Verification items for the finished model (mm, model axes). Round coordinates to 2 decimals unless told otherwise and drop trailing zeros. Write each loop counter-clockwise with the first axis right and the second up, starting at its lowest first coordinate (ties: lowest second). Pieces come first, ordered by that corner, then holes. Notation, with made-up numbers: (-5, 3) - (25, 3) arc R16 ccw to (25, 11) - close; hole circle Ø6 at (-19.5, -27.5). An arc over 180 degrees is marked (long way). Answer as a JSON object with one key per item and string values. Group by question number.
1) Section check C-C (z = 16.5). Enter the section's corners in (x, y).
2) Section check B-B (x = 0). Enter the section's corners in (y, z).
3) Go/stop test with flat-tipped pins: pin 1 Ø1.8 at (x, z) = (12.73, 12.73) entering from -Y; pin 2 Ø0.8 at (y, z) = (0.5, 9.5) entering from -X; pin 3 Ø0.8 at (y, z) = (0.5, 11) entering from +X; pin 4 Ø3.5 at (x, z) = (-4.66, 17.39) entering from +Y. Record where each tip stops, or that it passes through.
4) Section check A-A (z = 0). Enter the section's corners in (x, y), then the cut area to 3 significant figures.
5) Thickness scan on line 1 (Z direction, x = -0.5, y = 1.2); line 2 (X direction, y = 0.2, z = -11.5); line 3 (X direction, y = 1.2, z = -8.5). Record the ranges inside material, lowest first.
```python
from build123d import *

# Parameters (mm, degrees)
SKETCH1_R           = 21
SKETCH1_R_2         = 1.5
SKETCH1_R_3         = 4.4
BOSS_EXTRUDE1_DEPTH = 1.5


with BuildPart() as part:
    # Sketch1 → Boss-Extrude1 (new body)
    with BuildSketch(Plane(origin=(0, 0, 0), x_dir=(1, 0, 0), z_dir=(0, 1, 0))):
        with Locations(Location((0, 0, 0), (0, 0, 270))):
            Circle(SKETCH1_R)
        with Locations(Location((-8, 0, 0), (0, 0, 270))):
            Circle(SKETCH1_R_2, mode=Mode.SUBTRACT)
        with Locations(Location((8, 0, 0), (0, 0, 270))):
            Circle(SKETCH1_R_2, mode=Mode.SUBTRACT)
        with Locations(Location((0, 9.5, 0), (0, 0, 270))):
            Circle(SKETCH1_R_2, mode=Mode.SUBTRACT)
        with Locations(Location((0, -9.5, 0), (0, 0, 270))):
            Circle(SKETCH1_R_2, mode=Mode.SUBTRACT)
        with Locations(Location((-12.727922061, 12.727922061, 0), (0, 0, 270))):
            Circle(SKETCH1_R_2, mode=Mode.SUBTRACT)
        with Locations(Location((4.658742812, 17.386664873, 0), (0, 0, 270))):
            Circle(SKETCH1_R_2, mode=Mode.SUBTRACT)
        with Locations(Location((17.386664873, 4.658742812, 0), (0, 0, 270))):
            Circle(SKETCH1_R_2, mode=Mode.SUBTRACT)
        with Locations(Location((12.727922061, -12.727922061, 0), (0, 0, 270))):
            Circle(SKETCH1_R_2, mode=Mode.SUBTRACT)
        with Locations(Location((-4.658742812, -17.386664873, 0), (0, 0, 270))):
            Circle(SKETCH1_R_2, mode=Mode.SUBTRACT)
        with Locations(Location((0, 0, 0), (0, 0, 270))):
            Circle(SKETCH1_R_3, mode=Mode.SUBTRACT)
        with Locations(Location((-17.386664873, -4.658742812, 0), (0, 0, 270))):
            Circle(SKETCH1_R_2, mode=Mode.SUBTRACT)
        with BuildLine():
            Line((-8.660254038, 3), (-12, 3))
            ThreePointArc((-12, 3), (-13.664100589, 3.890599608), (-13.846153846, 5.769230769))
            ThreePointArc((-13.846153846, 5.769230769), (-10.606601718, 10.606601718), (-5.769230769, 13.846153846))
            ThreePointArc((-5.769230769, 13.846153846), (-3.890599608, 13.664100589), (-3, 12))
            Line((-3, 12), (-3, 8.660254038))
            ThreePointArc((-3, 8.660254038), (-3.267949192, 7.660254038), (-4, 6.92820323))
            ThreePointArc((-4, 6.92820323), (-5.656854249, 5.656854249), (-6.92820323, 4))
            ThreePointArc((-6.92820323, 4), (-7.660254038, 3.267949192), (-8.660254038, 3))
        make_face(mode=Mode.SUBTRACT)
        with BuildLine():
            Line((-8.660254038, -3), (-12, -3))
            ThreePointArc((-12, -3), (-13.664100589, -3.890599608), (-13.846153846, -5.769230769))
            ThreePointArc((-13.846153846, -5.769230769), (-10.606601718, -10.606601718), (-5.769230769, -13.846153846))
            ThreePointArc((-5.769230769, -13.846153846), (-3.890599608, -13.664100589), (-3, -12))
            Line((-3, -12), (-3, -8.660254038))
            ThreePointArc((-3, -8.660254038), (-3.267949192, -7.660254038), (-4, -6.92820323))
            ThreePointArc((-4, -6.92820323), (-5.656854249, -5.656854249), (-6.92820323, -4))
            ThreePointArc((-6.92820323, -4), (-7.660254038, -3.267949192), (-8.660254038, -3))
        make_face(mode=Mode.SUBTRACT)
        with BuildLine():
            Line((3, 8.660254038), (3, 12))
            ThreePointArc((3, 12), (3.890599608, 13.664100589), (5.769230769, 13.846153846))
            ThreePointArc((5.769230769, 13.846153846), (10.606601718, 10.606601718), (13.846153846, 5.769230769))
            ThreePointArc((13.846153846, 5.769230769), (13.664100589, 3.890599608), (12, 3))
            Line((12, 3), (8.660254038, 3))
            ThreePointArc((8.660254038, 3), (7.660254038, 3.267949192), (6.92820323, 4))
            ThreePointArc((6.92820323, 4), (5.656854249, 5.656854249), (4, 6.92820323))
            ThreePointArc((4, 6.92820323), (3.267949192, 7.660254038), (3, 8.660254038))
        make_face(mode=Mode.SUBTRACT)
        with BuildLine():
            Line((8.660254038, -3), (12, -3))
            ThreePointArc((12, -3), (13.664100589, -3.890599608), (13.846153846, -5.769230769))
            ThreePointArc((13.846153846, -5.769230769), (10.606601718, -10.606601718), (5.769230769, -13.846153846))
            ThreePointArc((5.769230769, -13.846153846), (3.890599608, -13.664100589), (3, -12))
            Line((3, -12), (3, -8.660254038))
            ThreePointArc((3, -8.660254038), (3.267949192, -7.660254038), (4, -6.92820323))
            ThreePointArc((4, -6.92820323), (5.656854249, -5.656854249), (6.92820323, -4))
            ThreePointArc((6.92820323, -4), (7.660254038, -3.267949192), (8.660254038, -3))
        make_face(mode=Mode.SUBTRACT)
    extrude(amount=BOSS_EXTRUDE1_DEPTH)


solid = part.part
```
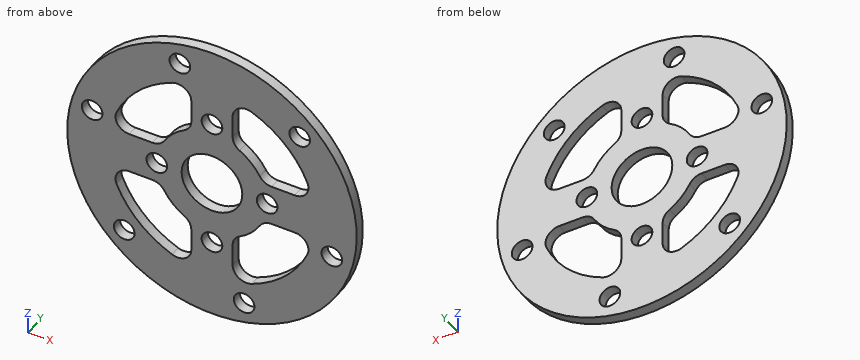
Returned:
{
 "1": {"outline": "(-12.99, 0) - (-5.87, 0) - (-5.87, 1.5) - (-12.99, 1.5) - close; (-3.45, 0) - (12.99, 0) - (12.99, 1.5) - (-3.45, 1.5) - close"},
 "2": {"outline": "(0, -21) - (1.5, -21) - (1.5, -11) - (0, -11) - close; (0, -8) - (1.5, -8) - (1.5, -4.4) - (0, -4.4) - close; (0, 4.4) - (1.5, 4.4) - (1.5, 8) - (0, 8) - close; (0, 11) - (1.5, 11) - (1.5, 21) - (0, 21) - close"},
 "3": {"pin 1": "through", "pin 2": "x = -18.93", "pin 3": "x = 18.13", "pin 4": "y = 1.5"},
 "4": {"outline": "(-21, 0) - (-9.5, 0) - (-9.5, 1.5) - (-21, 1.5) - close; (-6.5, 0) - (-4.4, 0) - (-4.4, 1.5) - (-6.5, 1.5) - close; (4.4, 0) - (6.5, 0) - (6.5, 1.5) - (4.4, 1.5) - close; (9.5, 0) - (21, 0) - (21, 1.5) - (9.5, 1.5) - close", "area": "40.8 mm2"},
 "5": {"line 1": "-20.99 to -10.91, -8.09 to -4.37, 4.37 to 8.09, 10.91 to 20.99", "line 2": "-17.57 to -13.59, -11.87 to -9.63, -3 to 3, 9.63 to 17.57", "line 3": "-19.2 to -12.36, -3.01 to -1.12, 1.12 to 3.01, 12.36 to 19.2"}
}
